CAD build for the part. Positions are in the model's coordinates, mm. Round coordinates to 2 decimals unless told otherwise and drop trailing zeros. Write each loop counter-clockwise with the first axis right and the second up, starting at its lowest first coordinate (ties: lowest second). Pieces come first, ordered by that corner, then holes. Notation, with made-up numbers: M -20,-21 L 21,-21 A11 ccw 21,-13 Z; hole C 66.25,40.25 d6. An arc over 180 degrees is marked long. Write each question's results on one line, items separated by ' | '. Start each with the question number.
```python
from build123d import *

# Parameters (mm, degrees)
BOSS_EXTRUDE1_OUTLINE_R   = 1.755
BOSS_EXTRUDE1_OUTLINE_R_2 = 8
BOSS_EXTRUDE1_DEPTH       = 3.175
BOSS_EXTRUDE2_START       = -3.175
SKETCH5_R                 = 7.95936
SKETCH5_R_2               = 1.71436
BOSS_EXTRUDE2_DEPTH       = 3.175


# Read off the part's stored shape, not the designer's step: Boss-Extrude1
with BuildPart() as part:
    # Boss-Extrude1 outline → Boss-Extrude1 (new body)
    with BuildSketch(Plane.XY):
        Polygon((-140, 10), (-140, -10), (-143.2, -10), (-143.2, -30), (-140, -30), (-140, -35.4), (-120, -35.4), (-120, -30), (-88, -30), (-88, -35.4), (-68, -35.4), (-68, -30), (-36, -30), (-36, -35.4), (-16, -35.4), (-16, -30), (16, -30), (16, -35.4), (36, -35.4), (36, -30), (68, -30), (68, -35.4), (88, -35.4), (88, -30), (120, -30), (120, -35.4), (140, -35.4), (140, -10), (143.2, -10), (143.2, 10), (140, 10), (140, 35.4), (120, 35.4), (120, 30), (88, 30), (88, 35.4), (68, 35.4), (68, 30), (36, 30), (36, 35.4), (16, 35.4), (16, 30), (-16, 30), (-16, 35.4), (-36, 35.4), (-36, 30), (-68, 30), (-68, 35.4), (-88, 35.4), (-88, 30), (-120, 30), (-120, 35.4), (-140, 35.4), (-140, 30), (-143.2, 30), (-143.2, 10), align=None)
        with Locations((-70, -15)):
            Circle(BOSS_EXTRUDE1_OUTLINE_R, mode=Mode.SUBTRACT)
        with BuildLine():
            ThreePointArc((22.474744871, -20.1), (23, -21.35), (22.474744871, -22.6))
            ThreePointArc((22.474744871, -22.6), (21.25, -25.6), (20.025255129, -22.6))
            ThreePointArc((20.025255129, -22.6), (19.5, -21.35), (20.025255129, -20.1))
            ThreePointArc((20.025255129, -20.1), (19.5, -18.85), (20.025255129, -17.6))
            ThreePointArc((20.025255129, -17.6), (19.5, -16.35), (20.025255129, -15.1))
            ThreePointArc((20.025255129, -15.1), (19.5, -13.85), (20.025255129, -12.6))
            ThreePointArc((20.025255129, -12.6), (19.5, -11.35), (20.025255129, -10.1))
            ThreePointArc((20.025255129, -10.1), (19.5, -8.85), (20.025255129, -7.6))
            ThreePointArc((20.025255129, -7.6), (19.5, -6.35), (20.025255129, -5.1))
            ThreePointArc((20.025255129, -5.1), (19.5, -3.85), (20.025255129, -2.6))
            ThreePointArc((20.025255129, -2.6), (19.5, -1.35), (20.025255129, -0.1))
            ThreePointArc((20.025255129, -0.1), (19.5, 1.15), (20.025255129, 2.4))
            ThreePointArc((20.025255129, 2.4), (19.5, 3.65), (20.025255129, 4.9))
            ThreePointArc((20.025255129, 4.9), (21.25, 7.9), (22.474744871, 4.9))
            ThreePointArc((22.474744871, 4.9), (23, 3.65), (22.474744871, 2.4))
            ThreePointArc((22.474744871, 2.4), (23, 1.15), (22.474744871, -0.1))
            ThreePointArc((22.474744871, -0.1), (23, -1.35), (22.474744871, -2.6))
            ThreePointArc((22.474744871, -2.6), (23, -3.85), (22.474744871, -5.1))
            ThreePointArc((22.474744871, -5.1), (23, -6.35), (22.474744871, -7.6))
            ThreePointArc((22.474744871, -7.6), (23, -8.85), (22.474744871, -10.1))
            ThreePointArc((22.474744871, -10.1), (23, -11.35), (22.474744871, -12.6))
            ThreePointArc((22.474744871, -12.6), (23, -13.85), (22.474744871, -15.1))
            ThreePointArc((22.474744871, -15.1), (23, -16.35), (22.474744871, -17.6))
            ThreePointArc((22.474744871, -17.6), (23, -18.85), (22.474744871, -20.1))
        make_face(mode=Mode.SUBTRACT)
        with Locations((112.5, -15)):
            Circle(BOSS_EXTRUDE1_OUTLINE_R, mode=Mode.SUBTRACT)
        with Locations((-60, 0)):
            Circle(BOSS_EXTRUDE1_OUTLINE_R_2, mode=Mode.SUBTRACT)
        with Locations((-70, 15)):
            Circle(BOSS_EXTRUDE1_OUTLINE_R, mode=Mode.SUBTRACT)
        with Locations((102.5, 0)):
            Circle(BOSS_EXTRUDE1_OUTLINE_R_2, mode=Mode.SUBTRACT)
        with Locations((112.5, 15)):
            Circle(BOSS_EXTRUDE1_OUTLINE_R, mode=Mode.SUBTRACT)
    extrude(amount=BOSS_EXTRUDE1_DEPTH)

    # Sketch5 → Boss-Extrude2 (add)
    with BuildSketch(Plane.XY.offset(3.175).offset(BOSS_EXTRUDE2_START)):
        Polygon((140.04064, 10.04064), (140.04064, 35.44064), (119.95936, 35.44064), (119.95936, 30.04064), (88.04064, 30.04064), (88.04064, 35.44064), (67.95936, 35.44064), (67.95936, 30.04064), (36.04064, 30.04064), (36.04064, 35.44064), (15.95936, 35.44064), (15.95936, 30.04064), (-15.95936, 30.04064), (-15.95936, 35.44064), (-36.04064, 35.44064), (-36.04064, 30.04064), (-67.95936, 30.04064), (-67.95936, 35.44064), (-88.04064, 35.44064), (-88.04064, 30.04064), (-119.95936, 30.04064), (-119.95936, 35.44064), (-140.04064, 35.44064), (-140.04064, 30.04064), (-143.24064, 30.04064), (-143.24064, 9.95936), (-140.04064, 9.95936), (-140.04064, -9.95936), (-143.24064, -9.95936), (-143.24064, -30.04064), (-140.04064, -30.04064), (-140.04064, -35.44064), (-119.95936, -35.44064), (-119.95936, -30.04064), (-88.04064, -30.04064), (-88.04064, -35.44064), (-67.95936, -35.44064), (-67.95936, -30.04064), (-36.04064, -30.04064), (-36.04064, -35.44064), (-15.95936, -35.44064), (-15.95936, -30.04064), (15.95936, -30.04064), (15.95936, -35.44064), (36.04064, -35.44064), (36.04064, -30.04064), (67.95936, -30.04064), (67.95936, -35.44064), (88.04064, -35.44064), (88.04064, -30.04064), (119.95936, -30.04064), (119.95936, -35.44064), (140.04064, -35.44064), (140.04064, -10.04064), (143.24064, -10.04064), (143.24064, 10.04064), align=None)
        with Locations((-60, 0)):
            Circle(SKETCH5_R, mode=Mode.SUBTRACT)
        with Locations((-70, 15)):
            Circle(SKETCH5_R_2, mode=Mode.SUBTRACT)
        with Locations((-70, -15)):
            Circle(SKETCH5_R_2, mode=Mode.SUBTRACT)
        with Locations((102.5, 0)):
            Circle(SKETCH5_R, mode=Mode.SUBTRACT)
        with Locations((112.5, 15)):
            Circle(SKETCH5_R_2, mode=Mode.SUBTRACT)
        with Locations((112.5, -15)):
            Circle(SKETCH5_R_2, mode=Mode.SUBTRACT)
        with BuildLine():
            ThreePointArc((22.474744871, 4.9), (21.25, 7.9), (20.025255129, 4.9))
            ThreePointArc((20.025255129, 4.9), (19.5, 3.65), (20.025255129, 2.4))
            ThreePointArc((20.025255129, 2.4), (19.5, 1.15), (20.025255129, -0.1))
            ThreePointArc((20.025255129, -0.1), (19.5, -1.35), (20.025255129, -2.6))
            ThreePointArc((20.025255129, -2.6), (19.5, -3.85), (20.025255129, -5.1))
            ThreePointArc((20.025255129, -5.1), (19.5, -6.35), (20.025255129, -7.6))
            ThreePointArc((20.025255129, -7.6), (19.5, -8.85), (20.025255129, -10.1))
            ThreePointArc((20.025255129, -10.1), (19.5, -11.35), (20.025255129, -12.6))
            ThreePointArc((20.025255129, -12.6), (19.5, -13.85), (20.025255129, -15.1))
            ThreePointArc((20.025255129, -15.1), (19.5, -16.35), (20.025255129, -17.6))
            ThreePointArc((20.025255129, -17.6), (19.5, -18.85), (20.025255129, -20.1))
            ThreePointArc((20.025255129, -20.1), (19.5, -21.35), (20.025255129, -22.6))
            ThreePointArc((20.025255129, -22.6), (21.25, -25.6), (22.474744871, -22.6))
            ThreePointArc((22.474744871, -22.6), (23, -21.35), (22.474744871, -20.1))
            ThreePointArc((22.474744871, -20.1), (23, -18.85), (22.474744871, -17.6))
            ThreePointArc((22.474744871, -17.6), (23, -16.35), (22.474744871, -15.1))
            ThreePointArc((22.474744871, -15.1), (23, -13.85), (22.474744871, -12.6))
            ThreePointArc((22.474744871, -12.6), (23, -11.35), (22.474744871, -10.1))
            ThreePointArc((22.474744871, -10.1), (23, -8.85), (22.474744871, -7.6))
            ThreePointArc((22.474744871, -7.6), (23, -6.35), (22.474744871, -5.1))
            ThreePointArc((22.474744871, -5.1), (23, -3.85), (22.474744871, -2.6))
            ThreePointArc((22.474744871, -2.6), (23, -1.35), (22.474744871, -0.1))
            ThreePointArc((22.474744871, -0.1), (23, 1.15), (22.474744871, 2.4))
            ThreePointArc((22.474744871, 2.4), (23, 3.65), (22.474744871, 4.9))
        make_face(mode=Mode.SUBTRACT)
    extrude(amount=BOSS_EXTRUDE2_DEPTH)


solid = part.part
```
1) Saw through at B-B, the plane z = 1.9. State how many separate pieces and enclosed holes the cut face has, plus the area to 3 significant figures.
2) Drop flat-ended pins along their axis: pin 1 Ø1 at (y, z) = (-33.5, 1) entering from +X; pin 2 Ø1.5 at (x, z) = (-58.5, 2.5) entering from -Y; pin 3 Ø1 at (x, z) = (103, 2) entering from +Y. Give the stop position or say it passes through.
3) Saw through at C-C, the plane x = -111. Write the cut outline in (y, z) (3 decimals).
4) Saw through at A-A, the plane x = -60. Write the cut outline in (y, z) (3 decimals).
5) Pull direction X, two halves, no side cores. Call faces 1 (the face through (-2, 0, 0)), 2 (the face through (-67.95, 0.35, 1.57)): pulls with the +X half, pulls with the -X half, needs draft (parallel to the pull), parting line crosses it, or undercut.
6) Wall check: line 1 along Y through (x, z) = (112.5, 1.1); line 2 along X through (y, z) = (-32, 0.45); line 3 along Y through (x, z) = (-70, 2.3). Give the ranges that are in metal, low to high. Write a range as from..to.
Filled sheet:
1) separate pieces: 1 | enclosed holes: 7 | area: 17,800 mm^2
2) pin 1: stops at x = 140.04 | pin 2: stops at y = -30.04 | pin 3: stops at y = 30.04
3) outline: M -30.041,0 L 30.041,0 L 30.041,3.175 L -30.041,3.175 Z
4) outline: M -30.041,0 L -7.959,0 L -7.959,3.175 L -30.041,3.175 Z; M 7.959,0 L 30.041,0 L 30.041,3.175 L 7.959,3.175 Z
5) face 1: needs draft | face 2: undercut
6) line 1: y = -30.04..-16.71, -13.29..13.29, 16.71..30.04 | line 2: x = -140.04..-119.96, -88.04..-67.96, -36.04..-15.96, 15.96..36.04, 67.96..88.04, 119.96..140.04 | line 3: y = -35.44..-16.71, -13.29..13.29, 16.71..35.44
